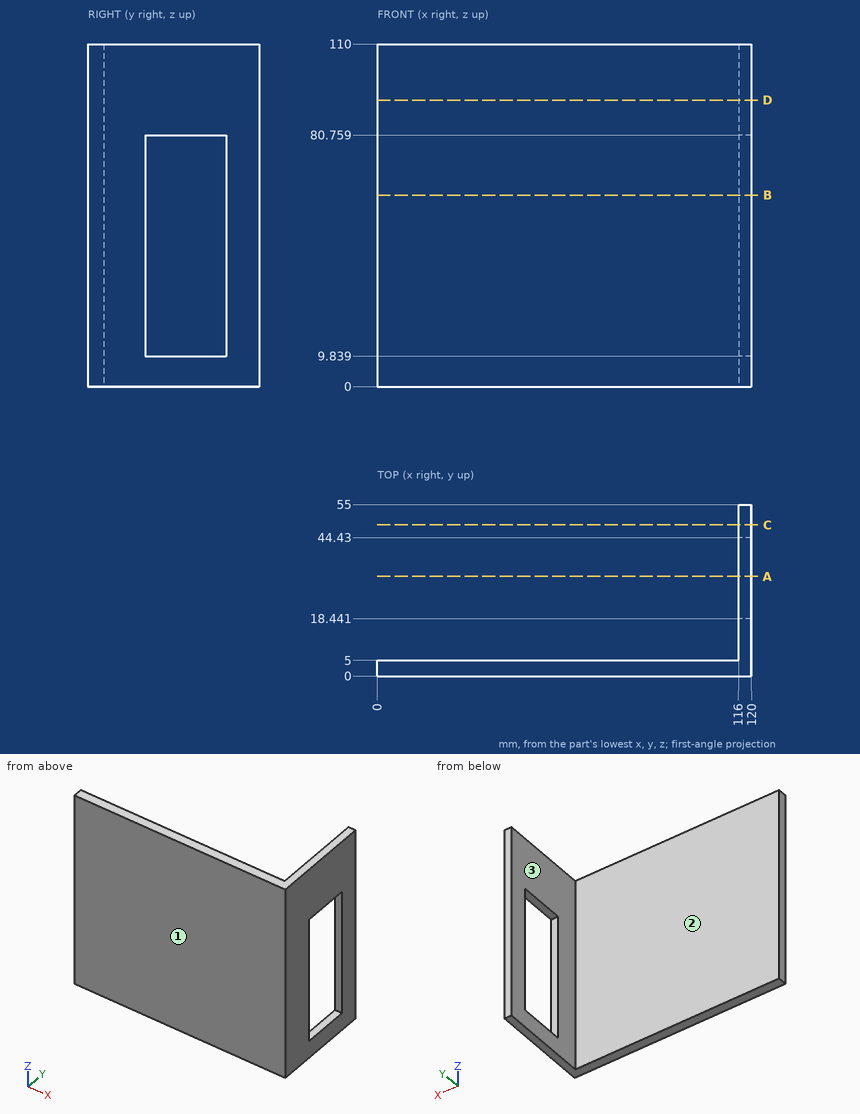
Study the drawing (mm; zero at the part's minimum x, y, z) and answer. Coordinates: 2 decimals unless noted, no trailing zeros. Write each loop counter-clockwise with the first axis right and the second up, starting at its lowest first coordinate (ties: lowest second). Pieces come first, ordered by that corner, then holes. Notation, with made-up numbers: M 85.25,-26.75 L 103.25,-26.75 A21 ccw 103.25,-21.75 Z; hole C 30,34.5 d4. An arc over 180 degrees is marked long. Use one line per item in the form item = value.
Item 1: Find section C-C, the plane y = 48.5. Give the vertices of the cut face in (x, z), plus the area to 3 significant figures.
Model answer:
outline = M 116,0 L 120,0 L 120,110 L 116,110 Z
area = 440 mm2
Item 2: Find the intervals of material crossed by probe 1 along Y at (x, z) = (103, 23); probe 2 along X at (y, z) = (15, 81), in increasing order.
Model answer:
probe_1 = 0 to 5
probe_2 = 116 to 120
Item 3: Find section D-D, the plane z = 92. Give the vertices of the cut face in (x, y).
Model answer:
outline = M 0,0 L 120,0 L 120,55 L 116,55 L 116,5 L 0,5 Z
Item 4: Find section A-A, the plane y = 32. Give the vertices of the cut face in (x, z).
Model answer:
outline = M 116,0 L 120,0 L 120,9.84 L 116,9.84 Z; M 116,80.76 L 120,80.76 L 120,110 L 116,110 Z
Item 5: Given P1, Ø3, axis at x = 96, z = 22, coming from the -Y side; P2, Ø10, axis at x = 83.5, z = 40, coming from the +Y side; P3, Ø15, axis at y = 37, z = 68, coming from the -X side, each flat-ended and moving along its own axis, determine where each tip first touches the part or whether it passes through.
Model answer:
P1 = 0
P2 = 5
P3 = 116
Item 6: The mould has two halves that part along Y. Classify the marked faces 1, 2 and 3: released by +Y, released by -Y, zero draft, split by the parting line, or undercut.
Model answer:
face_1 = released by -Y
face_2 = released by +Y
face_3 = zero draft
Item 7: Find section B-B, the plane z = 61.5. Give the vertices of the cut face in (x, y).
Model answer:
outline = M 0,0 L 120,0 L 120,18.44 L 116,18.44 L 116,5 L 0,5 Z; M 116,44.43 L 120,44.43 L 120,55 L 116,55 Z
